```python
from build123d import *

# Parameters (mm, degrees)
SKETCH1_W           = 6.5
SKETCH1_H           = 12.7
BOSS_EXTRUDE1_DEPTH = 5.0038
SKETCH2_W           = 3.2004
SKETCH2_H           = 3.4036
BOSS_EXTRUDE2_DEPTH = 5.0038
SKETCH3_W           = 3.2004
SKETCH3_H           = 4.5964
CUT_EXTRUDE1_DEPTH  = 1
CUT_EXTRUDE2_DEPTH  = 11
SKETCH5_R           = 0.4064
BOSS_EXTRUDE3_DEPTH = 3


with BuildPart() as part:
    # Sketch1 → Boss-Extrude1 (new body)
    with BuildSketch(Plane(origin=(0, 0, 0), x_dir=(1, 0, 0), z_dir=(0, 1, 0))):
        with Locations((-3.25, 6.35)):
            Rectangle(SKETCH1_W, SKETCH1_H)
    extrude(amount=BOSS_EXTRUDE1_DEPTH)

    # Sketch2 → Boss-Extrude2 (add)
    with BuildSketch(Plane(origin=(0, 5.0038, 0), x_dir=(1, 0, 0), z_dir=(0, 1, 0))):
        with Locations((-2.794, 3.363221349)):
            Rectangle(SKETCH2_W, SKETCH2_H)
    extrude(amount=BOSS_EXTRUDE2_DEPTH)

    # Sketch3 → Cut-Extrude1 (cut)
    with BuildSketch(Plane(origin=(0, 5.0038, 0), x_dir=(1, 0, 0), z_dir=(0, 1, 0))):
        with Locations((-2.794, 7.363221349)):
            Rectangle(SKETCH3_W, SKETCH3_H)
    extrude(amount=-CUT_EXTRUDE1_DEPTH, mode=Mode.SUBTRACT)

    # Sketch4 → Cut-Extrude2 (cut)
    with BuildSketch(Plane(origin=(-1.1938, 0, 0), x_dir=(0, 0, -1), z_dir=(1, 0, 0))):
        Polygon((1.661421349, 10.0076), (1.661421349, 9.45189334), (2.217128008, 10.0076), align=None)
        Polygon((3.271843346, 10.0076), (2.217128008, 10.0076), (2.772834668, 9.45189334), align=None)
        Polygon((4.38969876, 10.0076), (3.271843346, 10.0076), (3.890690082, 9.45189334), align=None)
        Polygon((5.065021349, 10.0076), (4.38969876, 10.0076), (5.065021349, 9.45189334), align=None)
    extrude(amount=-CUT_EXTRUDE2_DEPTH, mode=Mode.SUBTRACT)

    # Sketch5 → Boss-Extrude3 (add)
    with BuildSketch(Plane(origin=(0, 0, 0), x_dir=(-1, 0, 0), z_dir=(0, -1, 0))):
        with Locations(Location((2.794, 3, 0), (0, 0, 270))):
            Circle(SKETCH5_R)
        with Locations(Location((2.794, 5.5, 0), (0, 0, 270))):
            Circle(SKETCH5_R)
        with Locations(Location((2.794, 8, 0), (0, 0, 270))):
            Circle(SKETCH5_R)
    extrude(amount=BOSS_EXTRUDE3_DEPTH)


solid = part.part
```
The model under review builds one solid part; all positions refer to its coordinate system, in mm. A direction names the side the tool comes from. Give positions to 0.01 mm unless a question says otherwise; leave off trailing zeros. Write each loop counter-clockwise with the first axis right and the second up, starting at its lowest first coordinate (ties: lowest second). Pieces come first, ordered by that corner, then holes. Notation, with made-up numbers: (87, 59) -> (114, 59) arc R26 cw to (114, 96) -> close; hole circle Ø9 at (78, -2.75). An arc over 180 degrees is marked (long way). Answer in a Markdown table with one row per item.
1) Add section A-A on x = -4. State the section outline as (y, z) points, plus the area to 3 significant figures.
Worked answers:
| item | result |
|---|---|
| outline | (0, -12.7) -> (5, -12.7) -> (5, -9.66) -> (4, -9.66) -> (4, -5.07) -> (9.45, -5.07) -> (10.01, -4.39) -> (9.45, -3.89) -> (10.01, -3.27) -> (9.45, -2.77) -> (10.01, -2.22) -> (9.45, -1.66) -> (5, -1.66) -> (5, 0) -> (0, 0) -> close |
| area | 75.0 mm² |
2) Clearance check with flat-ended pins moving along their axes: P1, Ø0.5, axis at x = -3.5, y = 4.5, coming from the +Z side; P2, Ø2, axis at x = -5, z = -7.5, coming from the -Y side; P3, Ø2.5, axis at x = -3, z = -6.5, coming from the +Y side; P4, Ø1.5, axis at y = 8.5, z = -6.5, coming from the +X side. State where each tip first meets the part, or that it passes through.
Worked answers:
| item | result |
|---|---|
| P1 | z = 0 |
| P2 | y = 0 |
| P3 | y = 4 |
| P4 | through |
3) Add section B-B on z = -5.5. State the section outline as (x, y) points.
Worked answers:
| item | result |
|---|---|
| outline | (-6.5, 0) -> (-3.2, 0) -> (-3.2, -3) -> (-2.39, -3) -> (-2.39, 0) -> (0, 0) -> (0, 5) -> (-1.19, 5) -> (-1.19, 4) -> (-4.39, 4) -> (-4.39, 5) -> (-6.5, 5) -> close |
4) Tool access review of faces 4 (the flat face through (-4.394, 7, -3)), 5 (the flat face through (-1.194, 7, -3)), 6 (the flat face through (-3, 7, -1.661)), 7 (the flat face through (-1.194, 4.5, -7.3)), 8 (the cylindrical face through (-2.638, -1.479, -2.625)): name each direction out of +Z, -Z, +X, -X, +Y, -Y from which nothing blocks a thin tool from reaching the whole face with its end or side.
Worked answers:
| item | result |
|---|---|
| face 4 | +Z, -Z, -X, +Y |
| face 5 | +Z, -Z, +X, +Y |
| face 6 | +Z, +X, -X, +Y |
| face 7 | +Y |
| face 8 | -Y |
5) Mouldability with a two-part tool opening along X and no side actions: class faces 1 (the flat face through (-3.3, 0, -6.4)), 2 (the flat face through (-3, 4.004, -7)), 3 (the cylindrical face through (-2.547, -1.479, -8.323)) as +X half, -X half, draft (parallel to the pull), parting line (faces both ways), or undercut.
Worked answers:
| item | result |
|---|---|
| face 1 | draft |
| face 2 | undercut |
| face 3 | parting line |
6) For L1, parallel to Z at x = -2.5, y = -2; L2, parallel to Y at x = -1.25, z = -0.25; L3, parallel to Y at x = -3, z = -6.75, list the stretches that pass through material, from the lowest coordinate up. Write a range as [from, to].
Worked answers:
| item | result |
|---|---|
| L1 | [-8.28, -7.72], [-5.78, -5.22], [-3.28, -2.72] |
| L2 | [0, 5] |
| L3 | [0, 4] |
7) Add section C-C on y = 9. State the section outline as (x, z) points.
Worked answers:
| item | result |
|---|---|
| outline | (-4.39, -5.07) -> (-1.19, -5.07) -> (-1.19, -1.66) -> (-4.39, -1.66) -> close |
8) Add section D-D on z = -8.25. State the section outline as (x, y) points, plus the area to 3 significant figures.
Worked answers:
| item | result |
|---|---|
| outline | (-6.5, 0) -> (-3.11, 0) -> (-3.11, -3) -> (-2.47, -3) -> (-2.47, 0) -> (0, 0) -> (0, 5) -> (-1.19, 5) -> (-1.19, 4) -> (-4.39, 4) -> (-4.39, 5) -> (-6.5, 5) -> close |
| area | 31.2 mm² |
